The listing builds one solid part. Answer for the finished solid, in the listing's coordinates (mm). Face numbers are marked on the shaded views. A direction names the side the tool comes from. Give positions to 0.01 mm unless a question says otherwise; leave off trailing zeros. Loops run counter-clockwise (first coordinate to the right, second up) from the corner with the lowest first, then second, coordinate; pieces in that order, holes last.
Item 1: Section A-A, the plane z = 10 is taken. Give the vertices of the cut face in (x, y), and give its area (3 significant figures).
Item 2: Each of these flat-tipped pins is pushed along its axis until it touches: pin 1 Ø6 at (x, y) = (-9, -2.5) entering from +Z; pin 2 Ø5 at (x, z) = (0, 16.5) entering from +Y; pin 3 Ø4.5 at (x, z) = (-4, 10) entering from -Y. Where does it stop, or does it pass through?
Item 3: The mould has two halves that part along X. Classify the marked faces 3, 4, 5 and 6: pulls with the +X half, pulls with the -X half, needs draft (parallel to the pull), parting line crosses it, or undercut.
Item 4: Consider line 1 along X through (y, z) = (-3, 7.5); line 2 along Y through (x, z) = (1, 3.5); line 3 along Z through (x, y) = (-12.5, 10.5). Determine where each line is inside the solid, lowest interval first.
Item 5: Section B-B, the plane x = 4 is taken. Give the vertices of the cut face in (y, z).
Item 6: Section D-D, the plane z = 4 is taken. Give the vertices of the cut face in (x, y).
Item 7: Section C-C, the plane y = 16.5 is taken. Give the vertices of the cut face in (x, z).
Item 8: A tool of negligible diameter and unlimited length cuts with its end or side. For the marked faces 1 and 2, from which of +Z, -Z, +X, -X, +Y, -Y can it reach the whole face along a straight path? Write none if from no direction.
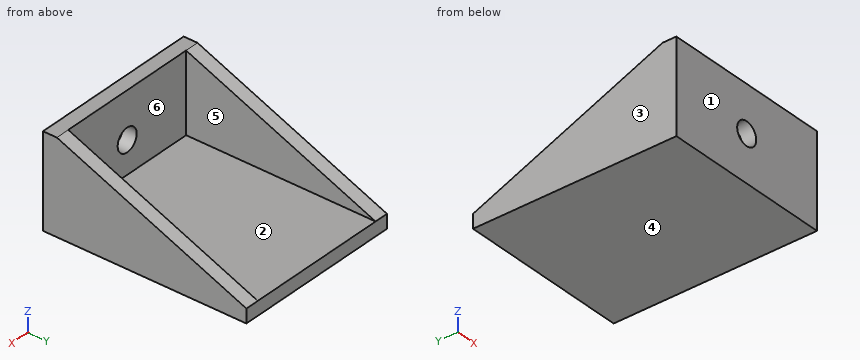
from build123d import *

# Parameters (mm, degrees)
F0_W     = 37
F0_H     = 44
F1_DEPTH = 3
F2_W     = 37
F2_H     = 17
F3_DEPTH = 3
F5_DEPTH = 3
F7_DEPTH = 3
F9_D     = 5


with BuildPart() as f1:
    # F0 (on Top) → F1 (new body)
    with BuildSketch(Plane.XY):
        with Locations((-3.996914, 0.254389)):
            Rectangle(F0_W, F0_H)
    extrude(amount=F1_DEPTH)

    # F2 (on face) → F3 (join)
    with BuildSketch(Plane.XZ.offset(21.745611)):
        with Locations((-3.996914, 11.5)):
            Rectangle(F2_W, F2_H)
    extrude(amount=-F3_DEPTH)

    # F4 (on face) → F5 (join)
    with BuildSketch(Plane.YZ.offset(14.503086)):
        Polygon((22.254389, 3), (-18.745611, 20), (-18.745611, 3), align=None)
    extrude(amount=-F5_DEPTH)

    # F6 (on face) → F7 (join)
    with BuildSketch(Plane(origin=(-22.496914, 0, 0), x_dir=(0, -1, 0), z_dir=(-1, 0, 0))):
        Polygon((18.745611, 3), (18.745611, 20), (-22.254389, 3), align=None)
    extrude(amount=-F7_DEPTH)

    # F9 (through all)
    with Locations(Plane.XZ.offset(21.745611)):
        with Locations((-3.996914, 10)):
            Hole(F9_D / 2)


solid = f1.part
Worked answers:
1. outline: (-22.5, -21.75) - (-6.5, -21.75) - (-6.5, -18.75) - (-19.5, -18.75) - (-19.5, 5.37) - (-22.5, 5.37) - close; (-1.5, -21.75) - (14.5, -21.75) - (14.5, 5.37) - (11.5, 5.37) - (11.5, -18.75) - (-1.5, -18.75) - close
1. area: 241 mm2
2. pin 1: stops at z = 3
2. pin 2: stops at y = -18.75
2. pin 3: passes through
3. face 3: pulls with the -X half
3. face 4: needs draft
3. face 5: undercut
3. face 6: undercut
4. line 1: x = -22.5 to -19.5, 11.5 to 14.5
4. line 2: y = -21.75 to -18.75
4. line 3: z = 0 to 3
5. outline: (-21.75, 0) - (22.25, 0) - (22.25, 3) - (-18.75, 3) - (-18.75, 20) - (-21.75, 20) - close
6. outline: (-22.5, -21.75) - (14.5, -21.75) - (14.5, 19.84) - (11.5, 19.84) - (11.5, -18.75) - (-19.5, -18.75) - (-19.5, 19.84) - (-22.5, 19.84) - close
7. outline: (-22.5, 0) - (14.5, 0) - (14.5, 5.39) - (11.5, 5.39) - (11.5, 3) - (-19.5, 3) - (-19.5, 5.39) - (-22.5, 5.39) - close
8. face 1: +Z, -Z, +X, -X, -Y
8. face 2: +Z, +Y
